from build123d import *

# Parameters (mm, degrees)
F0_W     = 25
F0_H     = 38
F0_W_2   = 22.9999984503
F0_H_2   = 15.5999984503
F0_H_3   = 7.7
F0_H_4   = 10.7
F1_DEPTH = 10
F2_W     = 25
F2_H     = 38
F2_W_2   = 22.9999984503
F2_H_2   = 15.5999984503
F2_H_3   = 7.7
F2_H_4   = 10.7
F3_DEPTH = 1
F4_DEPTH = 1
F5_W     = 23.0000000447
F5_H     = 9.0000000447
F6_DEPTH = 1


with BuildPart() as f1:
    # F0 (on Front) → F1 (new body)
    with BuildSketch(Plane.XZ):
        Rectangle(F0_W, F0_H)
        with Locations((0, -10.2)):
            Rectangle(F0_W_2, F0_H_2, mode=Mode.SUBTRACT)
        with Locations((0, 2.4499992251)):
            Rectangle(F0_W_2, F0_H_3, mode=Mode.SUBTRACT)
        with Locations((0, 12.6499992251)):
            Rectangle(F0_W_2, F0_H_4, mode=Mode.SUBTRACT)
    extrude(amount=F1_DEPTH)

    # F2 (on face) → F3 (join)
    with BuildSketch(Plane(origin=(0, 0, 0), x_dir=(-1, 0, 0), z_dir=(0, 1, 0))):
        Rectangle(F2_W, F2_H)
        with Locations((0, -10.2)):
            Rectangle(F2_W_2, F2_H_2, mode=Mode.SUBTRACT)
        with Locations((0, 2.4499992251)):
            Rectangle(F2_W_2, F2_H_3, mode=Mode.SUBTRACT)
        with Locations((0, 12.6499992251)):
            Rectangle(F2_W_2, F2_H_4, mode=Mode.SUBTRACT)
        with Locations((0, -10.2)):
            Rectangle(F2_W_2, F2_H_2)
        with Locations((0, 12.6499992251)):
            Rectangle(F2_W_2, F2_H_4)
        with Locations((0, 2.4499992251)):
            Rectangle(F2_W_2, F2_H_3)
    extrude(amount=F3_DEPTH)

    # F4 (add): a face of the model
    f4_faces = [f1.faces().sort_by_distance(p)[0] for p in [
        (0, -5, -17.9999992251),
    ]]
    extrude(f4_faces, amount=F4_DEPTH)

    # F5 (on face) → F6 (cut)
    with BuildSketch(Plane(origin=(0, 0, -19), x_dir=(1, 0, 0), z_dir=(0, 0, -1))):
        with Locations((0, 4.5)):
            Rectangle(F5_W, F5_H)
    extrude(amount=-F6_DEPTH, mode=Mode.SUBTRACT)


solid = f1.part
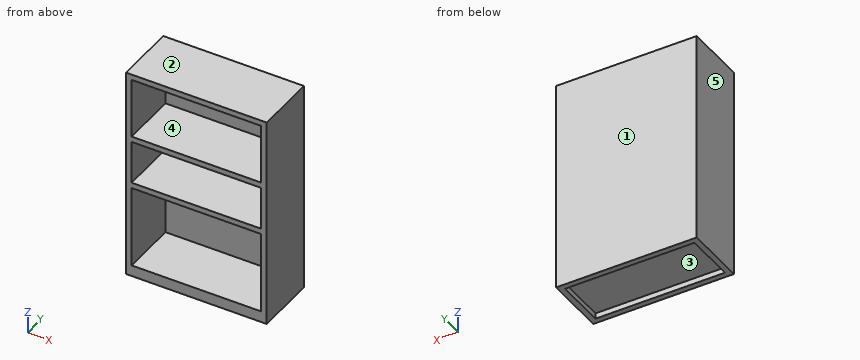
The listing builds one solid part. Answer for the finished solid, in the listing's coordinates (mm). Face numbers are marked on the shaded views. A direction names the side the tool comes from. Coordinates: 2 decimals unless noted, no trailing zeros. Loops run counter-clockwise (first coordinate to the right, second up) from the corner with the lowest first, then second, coordinate; pieces in that order, holes last. Notation, with made-up numbers: (4.5, -11.5) -> (56.5, -11.5) arc R28 ccw to (56.5, 26.5) -> close; hole circle Ø1 at (74, -20). An arc over 180 degrees is marked (long way). Write item = value, one per line. Start each with the question number.
1) Straight lines are drawn through the part: line 1 (Z direction, x = -1.5, y = -2.75); line 2 (X direction, y = -4.5, z = 1.5); line 3 (Y direction, x = 1, z = -16.5). For each, find the intervals that lie inside material, in ascending order. Write a range as from..to.
2) Given pin 1 Ø5 at (x, y) = (-5, -4) entering from -Z; pin 2 Ø4.5 at (x, z) = (1.5, -6.5) entering from -Y, each flat-ended and moving along its own axis, determine where each tip first touches the part or whether it passes through.
3) The mould has two halves that part along Y. Classify the marked faces 1, 2 and 3: released by +Y, released by -Y, zero draft, split by the parting line, or undercut.
4) A cutting plane is placed at B-B (y = -5.5). Give the vertices of the cut face in (x, z).
5) A cutting plane is placed at C-C (x = -10.75). Give the vertices of the cut face in (y, z).
6) A cutting plane is placed at A-A (z = 12.5). Give the vertices of the cut face in (x, y), then the cut area to 3 significant figures.
7) A tool of negligible diameter and unlimited length cuts with its end or side. For the marked faces 4 and 5, from which of +Z, -Z, +X, -X, +Y, -Y can it reach the whole face along a straight path? Write none if from no direction.
Responses:
q1.line_1 = -18..-17, -2.4..-1.4, 6.3..7.3, 18..19
q1.line_2 = -12.5..-11.5, 11.5..12.5
q1.line_3 = 0..1
q2.pin_1 = -18
q2.pin_2 = 0
q3.face_1 = released by +Y
q3.face_2 = zero draft
q3.face_3 = undercut
q4.outline = (-12.5, -19) -> (-11.5, -19) -> (-11.5, -18) -> (11.5, -18) -> (11.5, -19) -> (12.5, -19) -> (12.5, 19) -> (-12.5, 19) -> close; hole (-11.5, -17) -> (11.5, -17) -> (11.5, -2.4) -> (-11.5, -2.4) -> close; hole (-11.5, -1.4) -> (11.5, -1.4) -> (11.5, 6.3) -> (-11.5, 6.3) -> close; hole (-11.5, 7.3) -> (11.5, 7.3) -> (11.5, 18) -> (-11.5, 18) -> close
q5.outline = (-10, -19) -> (-9, -19) -> (-9, -18) -> (0, -18) -> (0, -19) -> (1, -19) -> (1, 19) -> (-10, 19) -> (-10, 18) -> (0, 18) -> (0, 7.3) -> (-10, 7.3) -> (-10, 6.3) -> (0, 6.3) -> (0, -1.4) -> (-10, -1.4) -> (-10, -2.4) -> (0, -2.4) -> (0, -17) -> (-10, -17) -> close
q6.outline = (-12.5, -10) -> (-11.5, -10) -> (-11.5, 0) -> (11.5, 0) -> (11.5, -10) -> (12.5, -10) -> (12.5, 1) -> (-12.5, 1) -> close
q6.area = 45.0 mm²
q7.face_4 = -Y
q7.face_5 = +Z, -Z, -X, +Y, -Y
